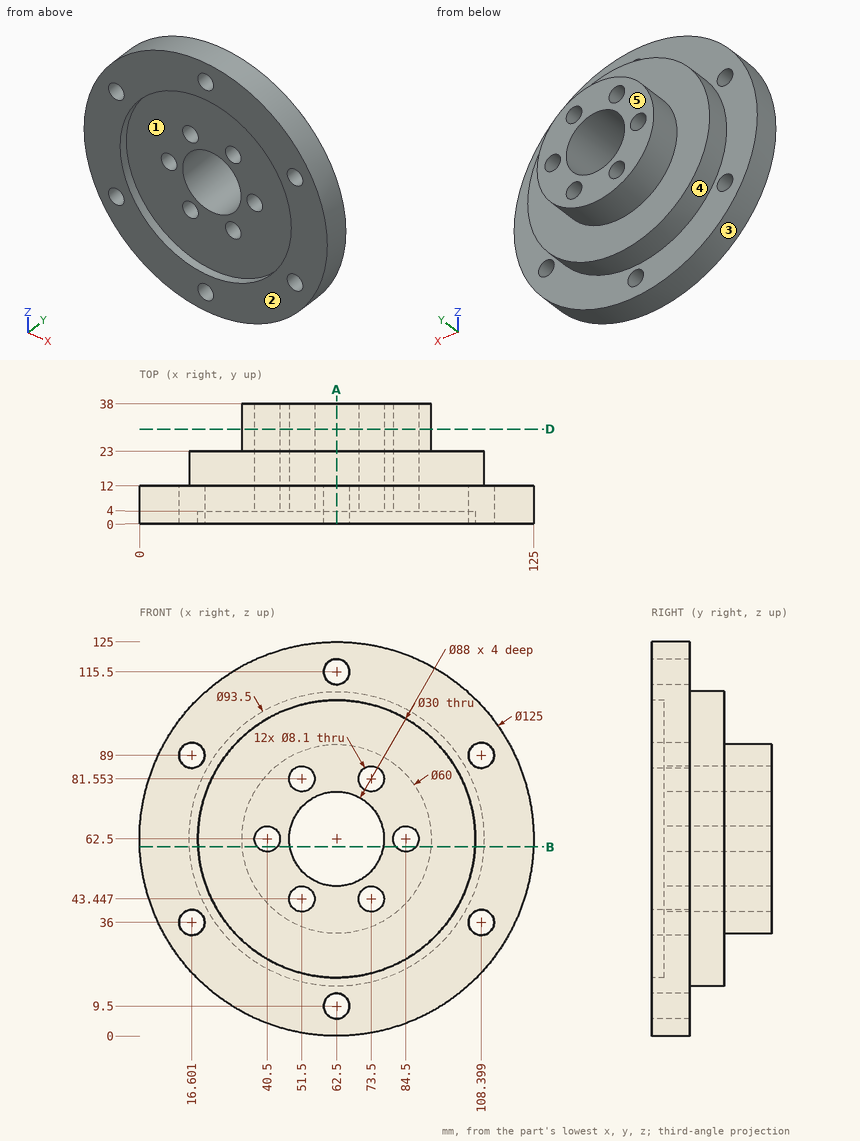
Here's the drawing with two shaded views (mm, measured from the low corner). I have some questions. A direction names the side the tool comes from. Give positions to 0.01 mm unless a question says otherwise; leave off trailing zeros. Loops run counter-clockwise (first coordinate to the right, second up) from the corner with the lowest first, then second, coordinate; pieces in that order, holes last. Notation, with made-up numbers: (81.25, 65.5) - (140.25, 65.5) arc R24 ccw to (140.25, 80.5) - close; hole circle Ø6 at (63, 80). An arc over 180 degrees is marked (long way). Answer in a Markdown table with one row per item. Add a question column.
Q1. If we section it at A-A (x = 62.5): List the corners of the cut face in (y, z) for me, plus the area to 3 significant figures.
Q2. If we section it at D-D (y = 30): List the corners of the cut face in (x, z) for me, plus the area to 3 significant figures.
Q3. Please list where these lines run through material, in increasing order: L1, parallel to Z at x = 62.5, y = 1; L2, parallel to Z at x = 62.5, y = 22.5; L3, parallel to X at y = 12.5, z = 61.5 (1 decimal). Write a range as from..to.
Q4. For pin 1 (6.5 mm diameter, centred on x = 51.5, z = 81.55, fed in from -Y); pin 2 (1.5 mm diameter, centred on x = 60.5, y = 8.5, fed in from -Z); pin 3 (13 mm diameter, centred on x = 16.6, z = 89, fed in from +Y); pin 4 (1.5 mm diameter, centred on x = 51.5, y = 19.5, fed in from +Z), each with a flat end and sliding along its axis, tell me the tip position at first contact or that it passes through.
Q5. We'd pull the mould along Z, two halves only. Please class the marked faces 1, 2 and 3: +Z half, -Z half, draft (parallel to the pull), parting line (faces both ways), or undercut.
Q6. If we section it at B-B (z = 60): State how many separate pieces and enclosed holes the cut face has, plus the area to 3 significant figures.
Q7. Which directions (+Z, -Z, +X, -X, +Y, -Y) give clear straight access to the entire face, cutting with the end or side of a thin tool? Please do the marked faces 4 and 5.
The answers:
| question | item | result |
|---|---|---|
| 1 | outline | (0, 0) - (12, 0) - (12, 5.45) - (0, 5.45) - close; (0, 13.55) - (12, 13.55) - (12, 15.75) - (23, 15.75) - (23, 32.5) - (38, 32.5) - (38, 47.5) - (4, 47.5) - (4, 18.5) - (0, 18.5) - close; (0, 106.5) - (4, 106.5) - (4, 77.5) - (38, 77.5) - (38, 92.5) - (23, 92.5) - (23, 109.25) - (12, 109.25) - (12, 111.45) - (0, 111.45) - close; (0, 119.55) - (12, 119.55) - (12, 125) - (0, 125) - close |
| 1 | area | 1,860 mm^2 |
| 2 | outline | circle Ø60 at (62.5, 62.5); hole circle Ø8.1 at (40.5, 62.5); hole circle Ø8.1 at (51.5, 43.45); hole circle Ø8.1 at (51.5, 81.55); hole circle Ø30 at (62.5, 62.5); hole circle Ø8.1 at (73.5, 43.45); hole circle Ø8.1 at (73.5, 81.55); hole circle Ø8.1 at (84.5, 62.5) |
| 2 | area | 1,810 mm^2 |
| 3 | L1 | z = 0..5.45, 13.55..18.5, 106.5..111.45, 119.55..125 |
| 3 | L2 | z = 15.75..47.5, 77.5..109.25 |
| 3 | L3 | x = 15.8..36.6, 44.4..47.5, 77.5..80.6, 88.4..109.2 |
| 4 | pin 1 | passes through |
| 4 | pin 2 | stops at z = 0.01 |
| 4 | pin 3 | stops at y = 23 |
| 4 | pin 4 | stops at z = 108.11 |
| 5 | face 1 | undercut |
| 5 | face 2 | draft |
| 5 | face 3 | parting line |
| 6 | separate pieces | 4 |
| 6 | enclosed holes | 0 |
| 6 | area | 1,630 mm^2 |
| 7 | face 4 | +Y |
| 7 | face 5 | +Z, -Z, +X, -X, +Y |
